Here's how the part is built. I have some questions about the finished solid (model axes, mm). Face numbers are marked on the shaded views. Round coordinates to 2 decimals unless told otherwise and drop trailing zeros. Loops run counter-clockwise (first coordinate to the right, second up) from the corner with the lowest first, then second, coordinate; pieces in that order, holes last. Notation, with made-up numbers: M 34.25,50 L 90.25,50 A34 cw 90.25,81 Z; hole C -27.5,-2.5 d6. An arc over 180 degrees is marked long. Use a Markdown table: item, result.
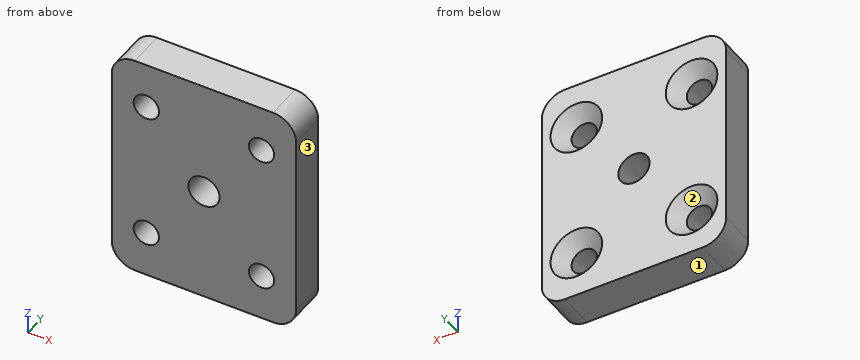
from build123d import *

# Parameters (mm, degrees)
SKETCH1_W                                            = 40
SKETCH1_H                                            = 50
BOSS_EXTRUDE1_DEPTH                                  = 8
CSK_FOR_M5_HEX_SOCKET_COUNTERSUNK_CAP_SC_D           = 5.5
CSK_FOR_M5_HEX_SOCKET_COUNTERSUNK_CAP_SC_CSINK_D     = 11.2
CSK_FOR_M5_HEX_SOCKET_COUNTERSUNK_CAP_SC_CSINK_ANGLE = 90
M8_TAPPED_HOLE1_D                                    = 6.8
FILLET1_R                                            = 5


with BuildPart() as part:
    # Sketch1 → Boss-Extrude1 (new body)
    with BuildSketch(Plane(origin=(0, 0, 0), x_dir=(1, 0, 0), z_dir=(0, 1, 0))):
        Rectangle(SKETCH1_W, SKETCH1_H)
    extrude(amount=BOSS_EXTRUDE1_DEPTH)

    # CSK for M5 Hex Socket Countersunk Cap Screw1 (through all)
    with Locations(Plane(origin=(0, 8, 0), x_dir=(1, 0, 0), z_dir=(0, 1, 0))):
        with Locations((-12.5, 15), (-12.5, -15), (12.5, -15), (12.5, 15)):
            CounterSinkHole(CSK_FOR_M5_HEX_SOCKET_COUNTERSUNK_CAP_SC_D / 2, CSK_FOR_M5_HEX_SOCKET_COUNTERSUNK_CAP_SC_CSINK_D / 2, counter_sink_angle=CSK_FOR_M5_HEX_SOCKET_COUNTERSUNK_CAP_SC_CSINK_ANGLE)

    # M8 Tapped Hole1 (through all)
    with Locations(Plane(origin=(0, 8, 0), x_dir=(1, 0, 0), z_dir=(0, 1, 0))):
        with Locations((0, 0)):
            Hole(M8_TAPPED_HOLE1_D / 2)

    # Fillet1
    fillet1_edges = [part.edges().sort_by_distance(p)[0] for p in [
        (20, 4, 25),
        (-20, 4, 25),
        (-20, 4, -25),
        (20, 4, -25),
    ]]
    fillet(fillet1_edges, radius=FILLET1_R)


solid = part.part
1. Imagine slicing it at A-A, the plane x = -12.5. Write out the boundary of the cut face in (y, z).
Answer sheet:
| item | result |
|---|---|
| outline | M 0,-25 L 8,-25 L 8,-20.6 L 5.15,-17.75 L 0,-17.75 Z; M 0,-12.25 L 5.15,-12.25 L 8,-9.4 L 8,9.4 L 5.15,12.25 L 0,12.25 Z; M 0,17.75 L 5.15,17.75 L 8,20.6 L 8,25 L 0,25 Z |
2. I need wall thicknesses on probe 1 along Z at (x, y) = (-12.5, 2.6); probe 2 along X at (y, z) = (3.05, 15); probe 3 along X at (y, z) = (5.25, 15). Which ranges of each line are inside material? Lowest first, please. Write a range as from..to.
Answer sheet:
| item | result |
|---|---|
| probe 1 | -25..-17.75, -12.25..12.25, 17.75..25 |
| probe 2 | -20..-15.25, -9.75..9.75, 15.25..20 |
| probe 3 | -20..-15.35, -9.65..9.65, 15.35..20 |
3. For pin 1 Ø4.5 at (x, z) = (-12.5, -15) entering from +Y; pin 2 Ø9 at (x, z) = (12.5, -15) entering from +Y, each with a flat end and sliding along its axis, tell me the tip position at first contact or that it passes through.
Answer sheet:
| item | result |
|---|---|
| pin 1 | through |
| pin 2 | y = 6.9 |
4. Imagine slicing it at C-C, the plane y = 6.5. Write out the boundary of the cut face in (x, z), then the cut area to 3 significant figures.
Answer sheet:
| item | result |
|---|---|
| outline | M -20,-20 A5 ccw -15,-25 L 15,-25 A5 ccw 20,-20 L 20,20 A5 ccw 15,25 L -15,25 A5 ccw -20,20 Z; hole C -12.5,-15 d8.2; hole C -12.5,15 d8.2; hole C 0,0 d6.8; hole C 12.5,-15 d8.2; hole C 12.5,15 d8.2 |
| area | 1,730 mm2 |
5. Imagine slicing it at D-D, the plane z = 0. Write out the boundary of the cut face in (x, y).
Answer sheet:
| item | result |
|---|---|
| outline | M -20,0 L -3.4,0 L -3.4,8 L -20,8 Z; M 3.4,0 L 20,0 L 20,8 L 3.4,8 Z |
6. Imagine slicing it at B-B, the plane z = -15. Write out the boundary of the cut face in (x, y), then the cut area to 3 significant figures.
Answer sheet:
| item | result |
|---|---|
| outline | M -20,0 L -15.25,0 L -15.25,5.15 L -18.1,8 L -20,8 Z; M -9.75,0 L 9.75,0 L 9.75,5.15 L 6.9,8 L -6.9,8 L -9.75,5.15 Z; M 15.25,0 L 20,0 L 20,8 L 18.1,8 L 15.25,5.15 Z |
| area | 216 mm2 |
7. We'd pull the mould along Z, two halves only. Please class the marked faces 1, 2 and 3: +Z half, -Z half, draft (parallel to the pull), parting line (faces both ways), or undercut.
Answer sheet:
| item | result |
|---|---|
| face 1 | -Z half |
| face 2 | undercut |
| face 3 | draft |
